The figure shows three views and two pictorial views of one solid part (mm, origin at its lowest corner). Answer the questions. Coordinates: 2 decimals unless noted, no trailing zeros. Write each loop counter-clockwise with the first axis right and the second up, starting at its lowest first coordinate (ties: lowest second). Pieces come first, ordered by that corner, then holes.
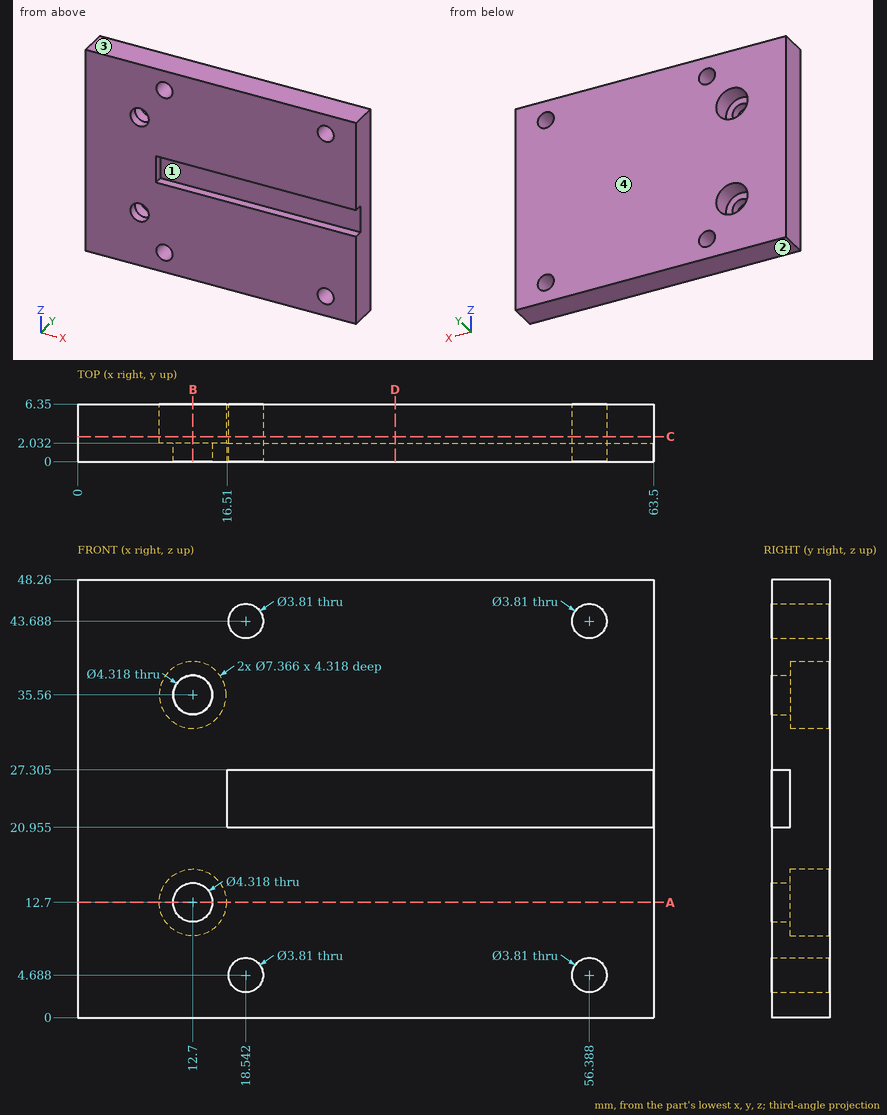
1. Flat-ended cylindrical pins translate along their axes: P1, Ø1, axis at y = 1, z = 23, coming from the +X side; P2, Ø2, axis at x = 11, z = 12, coming from the +Y side. Find the tip coordinate at first contact, or state that the pin passes through.
Results found:
P1: stops at x = 16.51
P2: stops at y = 2.03
2. Find the intervals of material crossed by L1, parallel to Z at x = 12.7, y = 1.5; L2, parallel to Z at x = 56.5, y = 0.75 (3 decimals); L3, parallel to X at y = 1.5, z = 35.56, in increasing order.
Results found:
L1: z = 0 to 10.54, 14.86 to 33.4, 37.72 to 48.26
L2: z = 0 to 2.786, 6.59 to 20.955, 27.305 to 41.786, 45.59 to 48.26
L3: x = 0 to 10.54, 14.86 to 63.5
3. Section A-A on z = 12.7 is taken. Give the vertices of the cut face in (x, y), then the cut area to 3 significant figures.
Results found:
outline: (0, 0) - (10.54, 0) - (10.54, 2.03) - (9.02, 2.03) - (9.02, 6.35) - (0, 6.35) - close; (14.86, 0) - (63.5, 0) - (63.5, 6.35) - (16.38, 6.35) - (16.38, 2.03) - (14.86, 2.03) - close
area: 363 mm2
4. For a pull along Z with two mould halves and no side action, classify the marked faces 1, 2, 3 and 4 as pulls with the +Z half, pulls with the -Z half, needs draft (parallel to the pull), parting line crosses it, or undercut.
Results found:
face 1: undercut
face 2: pulls with the -Z half
face 3: pulls with the +Z half
face 4: needs draft
5. Section B-B on x = 12.7 is taken. Give the vertices of the cut face in (y, z), then the cut area to 3 significant figures.
Results found:
outline: (0, 0) - (6.35, 0) - (6.35, 9.02) - (2.03, 9.02) - (2.03, 10.54) - (0, 10.54) - close; (0, 14.86) - (2.03, 14.86) - (2.03, 16.38) - (6.35, 16.38) - (6.35, 31.88) - (2.03, 31.88) - (2.03, 33.4) - (0, 33.4) - close; (0, 37.72) - (2.03, 37.72) - (2.03, 39.24) - (6.35, 39.24) - (6.35, 48.26) - (0, 48.26) - close
area: 225 mm2
6. Section D-D on x = 35 is taken. Give the vertices of the cut face in (y, z) (3 decimals), then the cut area to 3 significant figures.
Results found:
outline: (0, 0) - (6.35, 0) - (6.35, 48.26) - (0, 48.26) - (0, 27.305) - (2.032, 27.305) - (2.032, 20.955) - (0, 20.955) - close
area: 294 mm2
7. Section C-C on y = 2.75 is taken. Give the vertices of the cut face in (x, z) (3 decimals).
Results found:
outline: (0, 0) - (63.5, 0) - (63.5, 48.26) - (0, 48.26) - close; hole circle Ø7.366 at (12.7, 12.7); hole circle Ø7.366 at (12.7, 35.56); hole circle Ø3.81 at (18.542, 4.688); hole circle Ø3.81 at (18.542, 43.688); hole circle Ø3.81 at (56.388, 4.688); hole circle Ø3.81 at (56.388, 43.688)
